Build history of the part. All positions in model axes, mm. A direction names the side the tool comes from. Round coordinates to 2 decimals unless told otherwise and drop trailing zeros. Write each loop counter-clockwise with the first axis right and the second up, starting at its lowest first coordinate (ties: lowest second). Pieces come first, ordered by that corner, then holes. Notation, with made-up numbers: M 72.25,-2.75 L 127.25,-2.75 A33 cw 127.25,30.25 Z; hole C 22.5,25 d8. An arc over 180 degrees is marked long. One line per item, written item: value. Start each with the question number.
```python
from build123d import *

# Parameters (mm, degrees)
SKETCH1_W           = 22.098
SKETCH1_H           = 16.764
BOSS_EXTRUDE1_DEPTH = 1
SKETCH2_R           = 1
BOSS_EXTRUDE2_DEPTH = 1.1
SKETCH4_R           = 0.5
CUT_EXTRUDE1_DEPTH  = 1.1
SKETCH5_W           = 5.931061502
SKETCH5_H           = 5.124055134
BOSS_EXTRUDE3_DEPTH = 2
SKETCH6_W           = 5.112840458
SKETCH6_H           = 3.742927716
BOSS_EXTRUDE4_DEPTH = 1


with BuildPart() as part:
    # Sketch1 → Boss-Extrude1 (new body)
    with BuildSketch(Plane(origin=(0, 0, 0), x_dir=(1, 0, 0), z_dir=(0, 1, 0))):
        with Locations((11.049, 8.382)):
            Rectangle(SKETCH1_W, SKETCH1_H)
    extrude(amount=BOSS_EXTRUDE1_DEPTH)

    # Sketch2 → Boss-Extrude2 (add)
    with BuildSketch(Plane.XZ):
        with Locations((1.778, -14.984)):
            Circle(SKETCH2_R)
        with Locations((20.32, -14.985792546)):
            Circle(SKETCH2_R)
        with Locations((1.778, -12.444)):
            Circle(SKETCH2_R)
        with Locations((20.32, -12.444)):
            Circle(SKETCH2_R)
        with Locations((1.778, -1.78)):
            Circle(SKETCH2_R)
        with Locations((1.778, -4.32)):
            Circle(SKETCH2_R)
        with Locations((20.32, -4.32)):
            Circle(SKETCH2_R)
        with Locations((20.32, -1.78)):
            Circle(SKETCH2_R)
    extrude(amount=-BOSS_EXTRUDE2_DEPTH)

    # Sketch4 → Cut-Extrude1 (cut)
    with BuildSketch(Plane(origin=(0, 1.1, 0), x_dir=(1, 0, 0), z_dir=(0, 1, 0))):
        with Locations((1.778, 14.984)):
            Circle(SKETCH4_R)
        with Locations((1.778, 12.444)):
            Circle(SKETCH4_R)
        with Locations((1.778, 4.32)):
            Circle(SKETCH4_R)
        with Locations((1.778, 1.78)):
            Circle(SKETCH4_R)
        with Locations((20.32, 14.985792546)):
            Circle(SKETCH4_R)
        with Locations((20.32, 12.444)):
            Circle(SKETCH4_R)
        with Locations((20.32, 4.32)):
            Circle(SKETCH4_R)
        with Locations((20.32, 1.78)):
            Circle(SKETCH4_R)
    extrude(amount=-CUT_EXTRUDE1_DEPTH, mode=Mode.SUBTRACT)

    # Sketch5 → Boss-Extrude3 (add)
    with BuildSketch(Plane(origin=(0, 1, 0), x_dir=(1, 0, 0), z_dir=(0, 1, 0))):
        with Locations((14.107616891, 12.30880124)):
            Rectangle(SKETCH5_W, SKETCH5_H)
    extrude(amount=BOSS_EXTRUDE3_DEPTH)

    # Sketch6 → Boss-Extrude4 (add)
    with BuildSketch(Plane(origin=(0, 1, 0), x_dir=(1, 0, 0), z_dir=(0, 1, 0))):
        with Locations((7.742395479, 8.226436285)):
            Rectangle(SKETCH6_W, SKETCH6_H)
    extrude(amount=BOSS_EXTRUDE4_DEPTH)


solid = part.part
```
Item 1: Cut at A-A, the plane z = -1.78. Write the cut outline in (x, y).
Item 2: Cut at B-B, the plane x = 20.32. Count the separate pieces of the cut face and the enclosed holes in it, plus the area to 3 significant figures.
Item 3: Which spindle directions (+Z, -Z, +X, -X, +Y, -Y) get a long thin tool onto all of the face, cutting with end or side? Do faces 4 (the flat face through (21, 1.1, -12)), 5 (the flat face through (7.7, 1.5, -6.355)). Say none if no direction does.
Item 4: Drill centre lines: line 1 (X direction, y = 0.75, z = -1.78); line 2 (Z direction, x = 20.32, y = 0.85); line 3 (X direction, y = 0.55, z = -14.75). Where is each one in solid material? Low to high.
Item 5: Cut at C-C, the plane x = 7.75. Write the cut outline in (y, z).
Item 6: Drop flat-ended pins along their axis: pin 1 (1 mm diameter, centred on x = 1.5, z = -2, fed in from +Y); pin 2 (1.6 mm diameter, centred on y = 2, z = -11.5, fed in from -X); pin 3 (0.6 mm diameter, centred on x = 15, y = 1.5, fed in from +Z). Give the stop position or say it passes through.
Item 7: Two-plate mould, pull along Z, no slides. Class faces 1 (the flat face through (10.9, 0.5, -16.764)), 2 (the flat face through (8, 2, -8)), 3 (the cylindrical face through (2.24, 0.56, -14.79)): pulls with the +Z half, pulls with the -Z half, needs draft (parallel to the pull), parting line crosses it, or undercut.
Computed values:
1. outline: M 0,0 L 1.28,0 L 1.28,1.1 L 0.78,1.1 L 0.78,1 L 0,1 Z; M 2.28,0 L 19.82,0 L 19.82,1.1 L 19.32,1.1 L 19.32,1 L 2.78,1 L 2.78,1.1 L 2.28,1.1 Z; M 20.82,0 L 22.1,0 L 22.1,1 L 21.32,1 L 21.32,1.1 L 20.82,1.1 Z
2. separate pieces: 5
2. enclosed holes: 0
2. area: 13.2 mm2
3. face 4: +Z, -Z, +X, +Y
3. face 5: +Z, +X, -X, +Y
4. line 1: x = 0 to 1.28, 2.28 to 19.82, 20.82 to 22.1
4. line 2: z = -16.76 to -15.49, -14.49 to -12.94, -11.94 to -4.82, -3.82 to -2.28, -1.28 to 0
4. line 3: x = 0 to 1.34, 2.22 to 19.88, 20.76 to 22.1
5. outline: M 0,-16.76 L 1,-16.76 L 1,-10.1 L 2,-10.1 L 2,-6.35 L 1,-6.35 L 1,0 L 0,0 Z
6. pin 1: stops at y = 1.1
6. pin 2: stops at x = 11.14
6. pin 3: stops at z = -9.75
7. face 1: pulls with the -Z half
7. face 2: needs draft
7. face 3: undercut
